from build123d import *

# Parameters (mm, degrees)
F2_R = 5.08
F3_R = 1.137914


with BuildPart() as f1:
    # F0 (on Front) → F1 (revolve)
    with BuildSketch(Plane.XZ):
        Polygon((15.86405, 45.424398), (12.908017, 45.424398), (6.894663, 39.315261), (6.894663, -2.270045), (36.162157, -46.606813), (0, -46.606813), (0, -50.154049), (43.059569, -50.154049), (9.951984, 0), (9.951984, 39.315261), align=None)
    revolve(axis=Axis((0, 0, -48.380431), (0, 0, 1)))

    # F2
    f2_edges = [f1.edges().sort_by_distance(p)[0] for p in [
        (-43.059569, 0, -50.154049),
    ]]
    fillet(f2_edges, radius=F2_R)

    # F3
    f3_edges = [f1.edges().sort_by_distance(p)[0] for p in [
        (-15.86405, 0, 45.424398),
    ]]
    fillet(f3_edges, radius=F3_R)


solid = f1.part
Geometry: final body of the model. Coordinates: model frame, mm. A direction names the side the tool comes from. Give positions to 0.01 mm unless a question says otherwise; leave off trailing zeros. Loops run counter-clockwise (first coordinate to the right, second up) from the corner with the lowest first, then second, coordinate; pieces in that order, holes last. Notation, with made-up numbers: M 71.5,37.25 L 102.5,37.25 A27 cw 102.5,70.25 Z; hole C 35,54 d10. An arc over 180 degrees is marked long. Put each result on its own line as item: value. Start each with the question number.
1) Cut plane C-C (z = 18). Output: boundary loops of the cut face in (x, y).
2) Pull-direction query (X, two-part tool) for faces 3 (the flat face through (0, 0, -50.154)), 4 (the conical face through (-2.212, -9.962, 39.577)), 5 (the flat face through (-1, 1, -46.607)); classes: pulls with the +X half, pulls with the -X half, needs draft (parallel to the pull), parting line crosses it, or undercut.
3) Access query for faces 1 (the cylindrical face through (6.37, -2.64, 18.23)), 2 (the conical face through (-3, -15, -15)). Directions: +Z, -Z, +X, -X, +Y, -Y. A direction counts if a zero-diameter tool reaches every point of the face in a straight line with its end or side. Return the directions, or none.
4) Ray query, line 1 along Y through (x, z) = (0, 21.5); line 2 along Y through (x, z) = (-5, 8); line 3 along Z through (x, y) = (-16, -1). Return the intervals inside material, ascending.
5) Contact query for flat-ended pins moving along their axis: pin 1 (1 mm diameter, centred on x = -13.5, y = 5.5, fed in from +Z); pin 2 (8 mm diameter, centred on y = 6.5, z = -3, fed in from -X); pin 3 (10 mm diameter, centred on x = 6, z = -1.5, fed in from -Y). Output: stop coordinate, or through.
6) Cut plane D-D (z = -14.5). Output: boundary loops of the cut face in (x, y), then the cut area to 3 significant figures.
7) Cut plane A-A (y = 0). Output: boundary loops of the cut face in (x, z).
Verdict:
1. outline: C 0,0 d19.9; hole C 0,0 d13.79
2. face 3: needs draft
2. face 4: parting line crosses it
2. face 5: undercut
3. face 1: +Z
3. face 2: none
4. line 1: -9.95 to -6.89, 6.89 to 9.95
4. line 2: -8.6 to -4.75, 4.75 to 8.6
4. line 3: -50.15 to -46.61, -16.11 to -9.21
5. pin 1: z = 44.99
5. pin 2: x = -13.5
5. pin 3: y = -13.38
6. outline: C 0,0 d39.05; hole C 0,0 d29.94
6. area: 494 mm2
7. outline: M -37.86,-42.28 A5.08 ccw -33.62,-50.15 L 33.62,-50.15 A5.08 ccw 37.86,-42.28 L 9.95,0 L 9.95,39.32 L 14,43.5 A1.14 ccw 13.18,45.42 L 12.91,45.42 L 6.89,39.32 L 6.89,-2.27 L 36.16,-46.61 L -36.16,-46.61 L -6.89,-2.27 L -6.89,39.32 L -12.91,45.42 L -13.18,45.42 A1.14 ccw -14,43.5 L -9.95,39.32 L -9.95,0 Z
